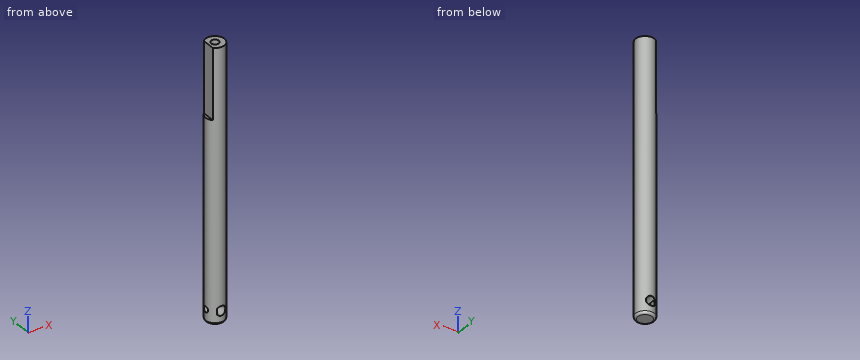
from build123d import *

# Parameters (mm, degrees)
SKETCH_3_R               = 4
EXTRUDE_2_DEPTH          = 57.5
CUT_EXTRUDE_1_DEPTH      = 58.777590812
CUT_EXTRUDE_1_DEPTH_BACK = 58.777590812
FILLET_1_R               = 1
M4X0_7_1_D               = 3.3
M4X0_7_1_DEPTH           = 10
M4X0_7_1_TIP             = 0.991420021
CUT_EXTRUDE_2_DEPTH      = 30


with BuildPart() as part:
    # 草图3 → 凸台-拉伸2 (new, symmetric)
    with BuildSketch(Plane.XY):
        Circle(SKETCH_3_R)
    extrude(amount=EXTRUDE_2_DEPTH, both=True)

    # 草图1 → 切除-拉伸1 (cut, two sides: drawn at the far end of the back side and taken through both)
    with BuildSketch(Plane(origin=(0, 0, 0), x_dir=(1, 0, 0), z_dir=(0, 1, 0)).offset(-CUT_EXTRUDE_1_DEPTH_BACK)):
        with BuildLine():
            Line((-1.625, 50.791695403), (-1.625, 53.208304597))
            ThreePointArc((-1.625, 53.208304597), (2.025, 52), (-1.625, 50.791695403))
        make_face()
    extrude(amount=CUT_EXTRUDE_1_DEPTH + CUT_EXTRUDE_1_DEPTH_BACK, mode=Mode.SUBTRACT)

    # 圆角1
    fillet_1_edges = [part.edges().sort_by_distance(p)[0] for p in [
        (-4, 0, -57.5),
    ]]
    fillet(fillet_1_edges, radius=FILLET_1_R)

    # M4x0.7 螺纹孔1
    with Locations(Plane.XY.offset(57.5)):
        with Locations((0, 0)):
            Hole(M4X0_7_1_D / 2, depth=M4X0_7_1_DEPTH)
            with Locations((0, 0, -(M4X0_7_1_DEPTH + M4X0_7_1_TIP / 2))):  # 118° drill point
                Cone(0, M4X0_7_1_D / 2, M4X0_7_1_TIP, mode=Mode.SUBTRACT)

    # 草图17 → M3x0.5 螺纹孔1 (revolve, cut)
    with BuildSketch(Plane(origin=(-1.625, 0, -52), x_dir=(0, 0, -1), z_dir=(0, 1, 0))):
        Polygon((0, 0), (0, 8.251075774), (1.25, 7.5), (1.25, 0), align=None)
    revolve(axis=Axis((4.725, 0, -52), (-1, 0, 0)), mode=Mode.SUBTRACT)

    # 草图13 → 切除-拉伸2 (cut)
    with BuildSketch(Plane.XY.offset(57.5)):
        with BuildLine():
            ThreePointArc((-2.828427125, 2.828427125), (-4, 0), (-2.828427125, -2.828427125))
            Line((-2.828427125, -2.828427125), (-2.828427125, 2.828427125))
        make_face()
    extrude(amount=-CUT_EXTRUDE_2_DEPTH, mode=Mode.SUBTRACT)


solid = part.part
Model file for the job. Use its own axes, mm. Coordinates: 2 decimals unless noted, no trailing zeros. Write each loop counter-clockwise with the first axis right and the second up, starting at its lowest first coordinate (ties: lowest second). Pieces come first, ordered by that corner, then holes. Notation, with made-up numbers: (9.5, 38) -> (24.5, 38) arc R16 cw to (24.5, 55) -> close; hole circle Ø5 at (83, -25.75). An arc over 180 degrees is marked (long way). One line per item, written item: value. Start each with the question number.
1) Probe probe 1 along Y at (x, z) = (0, 53.25); probe 2 along X at (y, z) = (0, 52.75); probe 3 along Z at (x, y) = (-1, -3.5). List the from-to ranges inside material, lowest first.
2) Flat gauge pins, fed straight in: pin 1 Ø1 at (x, z) = (-1, 17) entering from +Y; pin 2 Ø0.7 at (y, z) = (2.5, -52.5) entering from +X; pin 3 Ø0.9 at (x, y) = (-3.5, -1) entering from +Z. Where does each tip first touch, or does it go through?
3) Slice it at A-A on z = -52. Write the cut outline in (x, y) (3 decimals).
4) Slice it at B-B on z = -27. Write the cut outline in (x, y), then the cut area to 3 significant figures.
Answers follow:
1. probe 1: -4 to -1.65, 1.65 to 4
1. probe 2: -2.83 to -1.65, 1.65 to 4
1. probe 3: -57.27 to -53.76, -50.24 to 57.5
2. pin 1: y = 3.97
2. pin 2: x = 3.37
2. pin 3: z = 27.5
3. outline: (-3.8, -1.25) arc R4 ccw to (-1.625, -3.655) -> (-1.625, -1.25) -> close; (-3.8, 1.25) -> (-1.625, 1.25) -> (-1.625, 3.655) arc R4 ccw to start; (2.025, -3.45) arc R4 ccw to (2.025, 3.45) -> close
4. outline: circle Ø8 at (0, 0)
4. area: 50.3 mm2
